```python
from build123d import *

# Parameters (mm, degrees)
ESQUISSE1_W        = 155
ESQUISSE1_H        = 52
BOSS_EXTRU_1_DEPTH = 2
CONG_1_R           = 10
ESQUISSE2_R        = 11.9
BOSS_EXTRU_2_DEPTH = 6


with BuildPart() as part:
    # Esquisse1 → Boss.-Extru.1 (new body)
    with BuildSketch(Plane.XY):
        with Locations((29.422862753, 9.505149502)):
            Rectangle(ESQUISSE1_W, ESQUISSE1_H)
    extrude(amount=BOSS_EXTRU_1_DEPTH)

    # Congé1
    cong_1_edges = [part.edges().sort_by_distance(p)[0] for p in [
        (-48.077137247, 35.505149502, 1),
        (106.922862753, 35.505149502, 1),
        (106.922862753, -16.494850498, 1),
        (-48.077137247, -16.494850498, 1),
    ]]
    fillet(cong_1_edges, radius=CONG_1_R)

    # Esquisse2 → Boss.-Extru.2 (add)
    with BuildSketch(Plane.XY.offset(2)):
        with Locations((89.422862753, 9.375368795)):
            Circle(ESQUISSE2_R)
        with BuildLine():
            Line((-31.477137247, -8.024631205), (59.522862753, -8.024631205))
            ThreePointArc((59.522862753, -8.024631205), (61.573472418, -7.17524087), (62.422862753, -5.124631205))
            Line((62.422862753, -5.124631205), (62.422862753, 23.875368795))
            ThreePointArc((62.422862753, 23.875368795), (61.573472418, 25.925978461), (59.522862753, 26.775368795))
            Line((59.522862753, 26.775368795), (-31.477137247, 26.775368795))
            ThreePointArc((-31.477137247, 26.775368795), (-33.527746913, 25.925978461), (-34.377137247, 23.875368795))
            Line((-34.377137247, 23.875368795), (-34.377137247, -5.124631205))
            ThreePointArc((-34.377137247, -5.124631205), (-33.527746913, -7.17524087), (-31.477137247, -8.024631205))
        make_face()
    extrude(amount=BOSS_EXTRU_2_DEPTH)


solid = part.part
```
Geometry check sheet. Reference: the model listing, model coordinates, mm. A direction names the side the tool comes from. Round coordinates to 2 decimals unless told otherwise and drop trailing zeros. Loops run counter-clockwise (first coordinate to the right, second up) from the corner with the lowest first, then second, coordinate; pieces in that order, holes last. Notation, with made-up numbers: M -38,24 L -28,24 A29 cw -28,50 Z; hole C 3.25,-31.5 d10. An arc over 180 degrees is marked long. Return JSON: item names as keys, results as strings. Group by question number.
(1) Scan lines: line 1 along X through (y, z) = (9, 7.5); line 2 along Z through (x, y) = (83, -4); line 3 along Y through (x, z) = (0, 6). Record each from-to range of solid material in increasing order. Write a range as [from, to].
(2) Set-up check for faces 4 (the face through (-34.377, 10, 5)), 5 (the face through (28, 27, 2)), 6 (the face through (61.55, -7.2, 4.96)), 7 (the face through (-33.505, 25.948, 4.958)), 8 (the face through (-33.55, -7.15, 4.96)): record each of +Z, -Z, +X, -X, +Y, -Y from which the full face is reachable in a straight line by a thin tool's end or side.
(3) Section check C-C, the plane y = 0. Enter the section's corners in (x, z).
(4) Section check B-B, the plane x = 39.5. Enter the section's corners in (y, z), and give its area (3 significant figures).
(5) Section check D-D, the plane x = 82. Enter the section's corners in (y, z).
(6) Mould release check, pull along X, two halves, no side actions. Record for faces 1 (the face through (61.6, 25.9, 5)), 2 (the face through (-45.226, -13.488, 1.014)), 3 (the face through (62.423, 9, 5)): pulls with the +X half, pulls with the -X half, needs draft (parallel to the pull), parting line crosses it, or undercut.
(7) Go/stop test with flat-tipped pins: pin 1 (3 mm diameter, centred on y = 8.5, z = 6.5, fed in from -X); pin 2 (5 mm diameter, centred on x = 86.5, y = -6.5, fed in from +Z); pin 3 (1.5 mm diameter, centred on x = 50, z = 6.5, fed in from +Y). Record where each tip stops, or that it passes through.
(8) Section check A-A, the plane z = 4.25. Enter the section's corners in (x, y), and give its area (3 significant figures).
Data:
{
 "1": {"line 1": "[-34.38, 62.42], [77.53, 101.32]", "line 2": "[0, 2]", "line 3": "[-8.02, 26.78]"},
 "2": {"face 4": "+Z, -X, +Y, -Y", "face 5": "+Z", "face 6": "+Z, +X, -Y", "face 7": "+Z, -X, +Y", "face 8": "+Z, -X, -Y"},
 "3": {"outline": "M -48.08,0 L 106.92,0 L 106.92,2 L 96.75,2 L 96.75,8 L 82.09,8 L 82.09,2 L 62.42,2 L 62.42,8 L -34.38,8 L -34.38,2 L -48.08,2 Z"},
 "4": {"outline": "M -16.49,0 L 35.51,0 L 35.51,2 L 26.78,2 L 26.78,8 L -8.02,8 L -8.02,2 L -16.49,2 Z", "area": "313 mm²"},
 "5": {"outline": "M -16.49,0 L 35.51,0 L 35.51,2 L 18.68,2 L 18.68,8 L 0.07,8 L 0.07,2 L -16.49,2 Z"},
 "6": {"face 1": "pulls with the +X half", "face 2": "pulls with the -X half", "face 3": "undercut"},
 "7": {"pin 1": "x = -34.38", "pin 2": "z = 2", "pin 3": "y = 26.78"},
 "8": {"outline": "M -34.38,-5.12 A2.9 ccw -31.48,-8.02 L 59.52,-8.02 A2.9 ccw 62.42,-5.12 L 62.42,23.88 A2.9 ccw 59.52,26.78 L -31.48,26.78 A2.9 ccw -34.38,23.88 Z; C 89.42,9.38 d23.8", "area": "3,810 mm²"}
}
